Input: part model. Units: mm. Frame: model coordinates. Face numbers are marked on the shaded views. A direction names the side the tool comes from. Give positions to 0.01 mm unless a question says otherwise; leave off trailing zeros. Loops run counter-clockwise (first coordinate to the right, second up) from the corner with the lowest first, then second, coordinate; pieces in that order, holes last. Notation, with made-up numbers: M 27.5,-11.5 L 53.5,-11.5 A26 cw 53.5,5.5 Z; hole C -35.75,82 d8. An arc over 180 degrees is marked long. Answer as a JSON object with one key per item and string values. Group by question number.
1) Draft query along X for the marked faces 1, 2, 3 and 4. Return one class per face: +X half, -X half, draft (parallel to the pull), parting line (faces both ways), or undercut.
2) Ray query, L1, parallel to Y at x = 23.25, z = 1.6; L2, parallel to Y at x = 19, z = 0.65; L3, parallel to Y at x = -15.5, z = 4.55. Return the intervals inside material, ascending.
3) Section query D-D on x = 8.5. Return loops of the section in (y, z), plus the area to 3 significant figures.
4) Section query B-B on y = -7.5. Return loops of the section in (x, z).
5) First-contact query: P1, Ø10, axis at x = -11, y = 0.5, coming from the +Z side; P2, Ø2.5, axis at x = -8.65, y = 7.5, coming from the +Z side. Flat tips, straight axial feed; report the tip coordinate or a pass-through.
6) Access query for the marked faces 5, 6 and 7. Directions: +Z, -Z, +X, -X, +Y, -Y. A direction counts if a zero-diameter tool reaches every point of the face in a straight line with its end or side. Return the directions, or none.
7) Section query A-A on x = -8.65. Return loops of the section in (y, z), plus the area to 3 significant figures.
8) Section query C-C on y = 11.75. Return loops of the section in (x, z), plus the area to 3 significant figures.
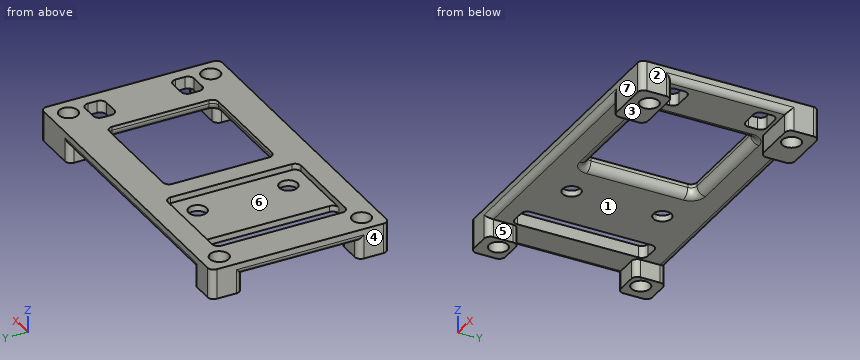
from build123d import *

# Parameters (mm, degrees)
SKETCH039_W     = 52.5
SKETCH039_H     = 29.5
SKETCH039_R     = 1.55
SKETCH039_R_2   = 1.5
SKETCH039_W_2   = 18.5
SKETCH039_H_2   = 18
SKETCH039_W_3   = 4
SKETCH039_H_3   = 22
SKETCH039_W_4   = 4.5
SKETCH039_H_4   = 3.5
PAD009_DEPTH    = 5
SKETCH040_W     = 11.65
SKETCH040_H     = 22
POCKET028_DEPTH = 1
POCKET029_DEPTH = 3
FILLET014_R     = 1
FILLET015_R     = 1.4


with BuildPart() as part:
    # Sketch039 → Pad009 (new body)
    with BuildSketch(Plane.XY):
        Rectangle(SKETCH039_W, SKETCH039_H)
        with Locations((-23.25, 11.75)):
            Circle(SKETCH039_R, mode=Mode.SUBTRACT)
        with Locations((23.25, 11.75)):
            Circle(SKETCH039_R, mode=Mode.SUBTRACT)
        with Locations((-23.25, -11.75)):
            Circle(SKETCH039_R, mode=Mode.SUBTRACT)
        with Locations((23.25, -11.75)):
            Circle(SKETCH039_R, mode=Mode.SUBTRACT)
        with Locations((-8.65, 7.5)):
            Circle(SKETCH039_R_2, mode=Mode.SUBTRACT)
        with Locations((-8.65, -7.5)):
            Circle(SKETCH039_R_2, mode=Mode.SUBTRACT)
        with Locations((7.5, 0)):
            Rectangle(SKETCH039_W_2, SKETCH039_H_2, mode=Mode.SUBTRACT)
        with Locations((-18.65, 0)):
            Rectangle(SKETCH039_W_3, SKETCH039_H_3, mode=Mode.SUBTRACT)
        with Locations((22, 7.25)):
            Rectangle(SKETCH039_W_4, SKETCH039_H_4, mode=Mode.SUBTRACT)
        with Locations((22, -7.25)):
            Rectangle(SKETCH039_W_4, SKETCH039_H_4, mode=Mode.SUBTRACT)
    extrude(amount=PAD009_DEPTH)

    # Sketch040 (on Face28 of Pad009) → Pocket028 (cut)
    with BuildSketch(Plane.XY.offset(5)):
        with Locations((-10.825, 0)):
            Rectangle(SKETCH040_W, SKETCH040_H)
    extrude(amount=-POCKET028_DEPTH, mode=Mode.SUBTRACT)

    # Sketch041 (on Face4 of Pocket028) → Pocket029 (cut)
    with BuildSketch(Plane(origin=(0, 0, 0), x_dir=(1, 0, 0), z_dir=(0, 0, -1))):
        Polygon((-21.05, 14.75), (-21.05, 9.55), (-26.25, 9.55), (-26.25, -9.55), (-21.05, -9.55), (-21.05, -14.75), (17.75, -14.75), (17.75, -9.55), (26.25, -9.55), (26.25, 9.55), (17.75, 9.55), (17.75, 14.75), align=None)
    extrude(amount=-POCKET029_DEPTH, mode=Mode.SUBTRACT)

    # Fillet014
    fillet014_edges = [part.edges().sort_by_distance(p)[0] for p in [
        (-26.25, -14.75, 2.5),
        (-26.25, 14.75, 2.5),
        (26.25, -14.75, 2.5),
        (17.75, -9.55, 1.5),
        (17.75, 9.55, 1.5),
        (-21.05, -9.55, 1.5),
        (-21.05, 9.55, 1.5),
        (26.25, 14.75, 2.5),
        (16.75, -9, 4),
        (-1.75, -9, 4),
        (16.75, 9, 4),
        (24.25, -5.5, 4),
        (24.25, 9, 4),
        (-16.65, 11, 3.5),
        (-20.65, -11, 4),
        (19.75, -9, 4),
        (19.75, 5.5, 4),
        (-20.65, 11, 4),
        (-1.75, 9, 4),
        (19.75, 9, 4),
        (19.75, -5.5, 4),
        (-16.65, -11, 3.5),
        (24.25, 5.5, 4),
        (24.25, -9, 4),
        (-5, -11, 4.5),
        (-5, 11, 4.5),
        (-21.05, -14.75, 1.5),
        (17.75, -14.75, 1.5),
        (26.25, -9.55, 1.5),
        (26.25, 9.55, 1.5),
        (-1.65, -14.75, 3),
        (17.75, 14.75, 1.5),
        (-21.05, 14.75, 1.5),
        (-26.25, -9.55, 1.5),
        (-26.25, 9.55, 1.5),
        (-26.25, 0, 3),
        (-1.65, 14.75, 3),
        (26.25, 0, 3),
    ]]
    fillet(fillet014_edges, radius=FILLET014_R)

    # Fillet015
    fillet015_edges = [part.edges().sort_by_distance(p)[0] for p in [
        (-1.75, 0, 3),
        (7.5, 9, 3),
        (16.75, 0, 3),
        (7.5, -9, 3),
    ]]
    fillet(fillet015_edges, radius=FILLET015_R)


solid = part.part
Output:
{
 "1": {"face 1": "undercut", "face 2": "+X half", "face 3": "draft", "face 4": "-X half"},
 "2": {"L1": "y = -14.75 to -13.3, -10.2 to -9.55, 9.55 to 10.2, 13.3 to 14.75", "L2": "y = -14.75 to -9.55, 9.55 to 14.75", "L3": "y = -14.75 to -11, 11 to 14.75"},
 "3": {"outline": "M -14.75,4 A1 ccw -13.75,3 L -10.4,3 A1.4 ccw -9,4.4 L -9,5 L -14.75,5 Z; M 9,4.4 A1.4 ccw 10.4,3 L 13.75,3 A1 ccw 14.75,4 L 14.75,5 L 9,5 Z", "area": "21.7 mm^2"},
 "4": {"outline": "M -26.25,4 A1 ccw -25.25,3 L -20.65,3 L -20.65,5 L -26.25,5 Z; M -16.65,3 L -10.15,3 L -10.15,4 L -16.65,4 Z; M -7.15,3 L -3.15,3 A1.4 ccw -1.75,4.4 L -1.75,5 L -5,5 L -5,4 L -7.15,4 Z; M 16.75,4.4 A1.4 ccw 18.15,3 L 19.75,3 L 19.75,5 L 16.75,5 Z; M 24.25,3 L 25.25,3 A1 ccw 26.25,4 L 26.25,5 L 24.25,5 Z"},
 "5": {"P1": "stops at z = 4", "P2": "passes through"},
 "6": {"face 5": "-Z, +Y, -Y", "face 6": "+Z", "face 7": "+Z, -Z, +X, -X, -Y"},
 "7": {"outline": "M -14.75,4 A1 ccw -13.75,3 L -9,3 L -9,4 L -11,4 L -11,5 L -14.75,5 Z; M -6,3 L 6,3 L 6,4 L -6,4 Z; M 9,3 L 13.75,3 A1 ccw 14.75,4 L 14.75,5 L 11,5 L 11,4 L 9,4 Z", "area": "30.6 mm^2"},
 "8": {"outline": "M -26.25,0 L -24.8,0 L -24.8,5 L -26.25,5 Z; M -21.7,0 L -21.05,0 L -21.05,3 L 17.75,3 L 17.75,0 L 21.7,0 L 21.7,5 L -21.7,5 Z; M 24.8,0 L 26.25,0 L 26.25,5 L 24.8,5 Z", "area": "115 mm^2"}
}
